```python
from build123d import *
from build123d.topology import SkipClean

# Parameters (mm, degrees)
CROQUIS1_R                   = 101.6
CROQUIS1_R_2                 = 7.9375
SALIENTE_EXTRUIR1_DEPTH      = 29
REDONDEO1_R                  = 28
CROQUIS2_R                   = 44.45
CORTAR_EXTRUIR1_DEPTH        = 8
CHAFL_N1_SIZE                = 15
CHAFL_N1_SIZE2               = 7.975641475
CHAFL_N2_SIZE                = 7.975641475
CHAFL_N2_SIZE_2              = 15
CORTAR_EXTRUIR2_DEPTH        = 147.581445076
CORTAR_EXTRUIR2_DEPTH_BACK   = 147.581445076
CROQUIS5_R                   = 7.9375
SALIENTE_EXTRUIR2_DEPTH      = 120
CROQUIS6_R                   = 12.9375
CROQUIS6_R_2                 = 7.9375
SALIENTE_EXTRUIR3_DEPTH      = 20
CROQUIS8_R                   = 3
CORTAR_EXTRUIR3_DEPTH        = 20
SALIENTE_EXTRUIR4_DEPTH      = 10
REDONDEO2_R                  = 1
CROQUIS11_R                  = 15
CORTAR_EXTRUIR4_DEPTH        = 50
SALIENTE_EXTRUIR5_DEPTH      = 5
SALIENTE_EXTRUIR5_DEPTH_BACK = 50
CROQUIS12_R                  = 15
CROQUIS12_R_2                = 7.9375
CROQUIS15_R                  = 7.9375
SALIENTE_EXTRUIR7_DEPTH      = 5
CROQUIS13_R                  = 3
SALIENTE_EXTRUIR8_DEPTH      = 5
SALIENTE_EXTRUIR8_2_DEPTH    = 5
SALIENTE_EXTRUIR8_3_DEPTH    = 5
SALIENTE_EXTRUIR8_4_DEPTH    = 5
CROQUIS17_R                  = 3
CORTAR_EXTRUIR5_DEPTH        = 16


with BuildPart() as part:
    # Croquis1 → Saliente-Extruir1 (new, symmetric)
    with BuildSketch(Plane.XY):
        with Locations(Location((0, 0, 0), (0, 0, 180))):
            Circle(CROQUIS1_R)
        with Locations(Location((0, 0, 0), (0, 0, 180))):
            Circle(CROQUIS1_R_2, mode=Mode.SUBTRACT)
    extrude(amount=SALIENTE_EXTRUIR1_DEPTH, both=True)

    # Redondeo1
    redondeo1_edges = [part.edges().sort_by_distance(p)[0] for p in [
        (101.6, 0, -29),
        (101.6, 0, 29),
    ]]
    fillet(redondeo1_edges, radius=REDONDEO1_R)

    # Croquis2 → Cortar-Extruir1 (cut)
    with BuildSketch(Plane(origin=(0, 0, -29), x_dir=(-1, 0, 0), z_dir=(0, 0, -1))):
        Circle(CROQUIS2_R)
    cortar_extruir1 = extrude(amount=-CORTAR_EXTRUIR1_DEPTH, mode=Mode.SUBTRACT)

    # Simetría3: Cortar-Extruir1 across plane
    add(cortar_extruir1.mirror(Plane.XY), mode=Mode.SUBTRACT)

    # Chaflán1
    chafl_n1_edges = [part.edges().sort_by_distance(p)[0] for p in [
        (44.45, 0, -29),
    ]]
    chafl_n1_side = [part.faces().sort_by_distance(p)[0] for p in [
        (71.518277636, 0, -29),
    ]]
    chamfer(chafl_n1_edges, length=CHAFL_N1_SIZE, length2=CHAFL_N1_SIZE2, reference=chafl_n1_side[0])

    # Chaflán2
    # the kernel refuses this chamfer: 15, 7.975641475 mm, written as the material it takes off along each edge
    with BuildSketch(Plane(origin=(0, 0, 29), x_dir=(-1, 0, 0), z_dir=(0, -1, 0))) as chafl_n2_piece_1_section:
        Polygon((44.45 + CHAFL_N2_SIZE, 0), (44.45, CHAFL_N2_SIZE_2), (44.45, 0), align=None)
    chafl_n2_piece_1 = revolve(axis=Axis((0, 0, 29), (0, 0, -1)), mode=Mode.PRIVATE)
    chafl_n2_piece_1 = split(chafl_n2_piece_1, bisect_by=Plane(origin=(50.219175815, 0, 21), z_dir=(0, 0, 1)), keep=Keep.TOP, mode=Mode.PRIVATE)
    add(chafl_n2_piece_1, mode=Mode.SUBTRACT)

    # Croquis3 → Cortar-Extruir2 (cut, two sides: drawn at the far end of the back side and taken through both)
    with BuildSketch(Plane(origin=(0, 0, 0), x_dir=(0, 0, -1), z_dir=(1, 0, 0)).offset(-CORTAR_EXTRUIR2_DEPTH_BACK)):
        Polygon((0, -580.951086966), (0, -121.331484358), (0, 121.331484358), (0, 580.951086966), (-919.239205217, 580.951086966), (-919.239205217, -580.951086966), align=None)
    extrude(amount=CORTAR_EXTRUIR2_DEPTH + CORTAR_EXTRUIR2_DEPTH_BACK, mode=Mode.SUBTRACT)

    # Simetría4: part across plane


with BuildPart() as part_1:
    add(part.part)
    add(part.part.mirror(Plane(origin=(376.375487344, -121.331484358, 0), x_dir=(1, 0, 0), z_dir=(0, 0, 1))))

    # Croquis11 → Cortar-Extruir4 (cut)
    with BuildSketch(Plane.XY.offset(21)):
        Circle(CROQUIS11_R)
    extrude(amount=-CORTAR_EXTRUIR4_DEPTH, mode=Mode.SUBTRACT)


with BuildPart() as body_2:
    # Croquis5 → Saliente-Extruir2 (new body)
    with BuildSketch(Plane.XY.offset(21)):
        with Locations(Location((0, 0, 0), (0, 0, 180))):
            Circle(CROQUIS5_R)
    extrude(amount=-SALIENTE_EXTRUIR2_DEPTH)


with BuildPart() as body_3:
    # Croquis6 → Saliente-Extruir3 (new body)
    with BuildSketch(Plane(origin=(0, 0, -99), x_dir=(-1, 0, 0), z_dir=(0, 0, -1))):
        Circle(CROQUIS6_R)
        Circle(CROQUIS6_R_2, mode=Mode.SUBTRACT)
    extrude(amount=-SALIENTE_EXTRUIR3_DEPTH)

    # Croquis8 → Cortar-Extruir3 (cut)
    with BuildSketch(Plane(origin=(0, 0, 0), x_dir=(1, 0, 0), z_dir=(0, 1, 0))):
        with Locations(Location((0, 89, 0), (0, 0, 90))):
            Circle(CROQUIS8_R)
    extrude(amount=CORTAR_EXTRUIR3_DEPTH, mode=Mode.SUBTRACT)

    # Croquis10 → Saliente-Extruir4 (add)
    with BuildSketch(Plane(origin=(0, 0, -99), x_dir=(-1, 0, 0), z_dir=(0, 0, -1))):
        with BuildLine():
            Line((-5, 17.5), (5, 17.5))
            ThreePointArc((5, 17.5), (7.856559563, 13.607960336), (12.655444566, 13.080127019))
            Line((12.655444566, 13.080127019), (17.655444566, 4.419872981))
            ThreePointArc((17.655444566, 4.419872981), (15.713119126, 0), (17.655444566, -4.419872981))
            Line((17.655444566, -4.419872981), (12.655444566, -13.080127019))
            ThreePointArc((12.655444566, -13.080127019), (7.856559563, -13.607960336), (5, -17.5))
            Line((5, -17.5), (-5, -17.5))
            ThreePointArc((-5, -17.5), (-7.856559563, -13.607960336), (-12.655444566, -13.080127019))
            Line((-12.655444566, -13.080127019), (-17.655444566, -4.419872981))
            ThreePointArc((-17.655444566, -4.419872981), (-15.713119126, 0), (-17.655444566, 4.419872981))
            Line((-17.655444566, 4.419872981), (-12.655444566, 13.080127019))
            ThreePointArc((-12.655444566, 13.080127019), (-7.856559563, 13.607960336), (-5, 17.5))
        make_face()
    extrude(amount=SALIENTE_EXTRUIR4_DEPTH)

    # Redondeo2
    redondeo2_edges = [body_3.edges().sort_by_distance(p)[0] for p in [
        (5, 17.5, -104),
        (12.655444566, 13.080127019, -104),
        (17.655444566, 4.419872981, -104),
        (17.655444566, -4.419872981, -104),
        (12.655444566, -13.080127019, -104),
        (5, -17.5, -104),
        (-5, -17.5, -104),
        (-12.655444566, -13.080127019, -104),
        (-17.655444566, -4.419872981, -104),
        (-17.655444566, 4.419872981, -104),
        (-12.655444566, 13.080127019, -104),
        (-5, 17.5, -104),
    ]]
    fillet(redondeo2_edges, radius=REDONDEO2_R)


with BuildPart() as body_4:
    # Croquis12 → Saliente-Extruir5 (new, two sides: drawn at the far end of the back side and taken through both)
    with BuildSketch(Plane.XY.offset(21).offset(-SALIENTE_EXTRUIR5_DEPTH_BACK)):
        Circle(CROQUIS12_R)
        with Locations(Location((0, 0, 0), (0, 0, 180))):
            Circle(CROQUIS12_R_2, mode=Mode.SUBTRACT)
    extrude(amount=SALIENTE_EXTRUIR5_DEPTH + SALIENTE_EXTRUIR5_DEPTH_BACK)


with BuildPart() as body_5:
    # Croquis15 → Saliente-Extruir7 (new body)
    with BuildSketch(Plane.XY.offset(21)):
        with Locations(Location((0, 0, 0), (0, 0, 180))):
            Circle(CROQUIS15_R)
    extrude(amount=SALIENTE_EXTRUIR7_DEPTH)

    # Combinar1: union body 2
    add(body_2.part)


with BuildPart() as body_5_2:
    # Croquis13 → Saliente-Extruir8 (new body)
    with BuildSketch(Plane.XY.offset(26)):
        with BuildLine():
            Line((5, -25), (5, -6.164730834))
            ThreePointArc((5, -6.164730834), (0, -7.9375), (-5, -6.164730834))
            Line((-5, -6.164730834), (-5, -25))
            Line((-5, -25), (5, -25))
        make_face()
        with Locations((0, -18.5)):
            Circle(CROQUIS13_R, mode=Mode.SUBTRACT)
    extrude(amount=-SALIENTE_EXTRUIR8_DEPTH)


with BuildPart() as body_6:
    # Croquis13 → Saliente-Extruir8 2 (new body)
    with BuildSketch(Plane.XY.offset(26)):
        with BuildLine():
            Line((-5, 25), (5, 25))
            Line((5, 25), (5, 6.164730834))
            ThreePointArc((5, 6.164730834), (0, 7.9375), (-5, 6.164730834))
            Line((-5, 6.164730834), (-5, 25))
        make_face()
        with Locations((0, 18.5)):
            Circle(CROQUIS13_R, mode=Mode.SUBTRACT)
    extrude(amount=-SALIENTE_EXTRUIR8_2_DEPTH)


with BuildPart() as body_7:
    # Croquis13 → Saliente-Extruir8 3 (new body)
    with BuildSketch(Plane.XY.offset(26)):
        with BuildLine():
            Line((-25, -5), (-6.164730834, -5))
            ThreePointArc((-6.164730834, -5), (-7.9375, 0), (-6.164730834, 5))
            Line((-6.164730834, 5), (-25, 5))
            Line((-25, 5), (-25, 0))
            Line((-25, 0), (-25, -5))
        make_face()
        with Locations((-18.5, 0)):
            Circle(CROQUIS13_R, mode=Mode.SUBTRACT)
    extrude(amount=-SALIENTE_EXTRUIR8_3_DEPTH)


with BuildPart() as body_8:
    # Croquis13 → Saliente-Extruir8 4 (new body)
    with BuildSketch(Plane.XY.offset(26)):
        with BuildLine():
            Line((25, -5), (25, 5))
            Line((25, 5), (6.164730834, 5))
            ThreePointArc((6.164730834, 5), (7.9375, 0), (6.164730834, -5))
            Line((6.164730834, -5), (25, -5))
        make_face()
        with Locations((18.5, 0)):
            Circle(CROQUIS13_R, mode=Mode.SUBTRACT)
    extrude(amount=-SALIENTE_EXTRUIR8_4_DEPTH)


with BuildPart() as body_4_1:
    add(body_4.part)

    # Combinar2: union body 6, body 8, body 5 2, body 7
    add(body_6.part)
    add(body_8.part)
    add(body_5_2.part)
    add(body_7.part)

    # Croquis17 → Cortar-Extruir5 (cut)
    with SkipClean():  # the faces are left unmerged after this step: merging them gives an invalid solid
        with BuildSketch(Plane(origin=(0, 0, 0), x_dir=(1, 0, 0), z_dir=(0, 1, 0))):
            with Locations(Location((0, 24, 0), (0, 0, 90))):
                Circle(CROQUIS17_R)
        extrude(amount=CORTAR_EXTRUIR5_DEPTH, mode=Mode.SUBTRACT)


solid = part_1.part
```
Model file for the job. Use its own axes, mm. A direction names the side the tool comes from. Coordinates: 2 decimals unless noted, no trailing zeros. Loops run counter-clockwise (first coordinate to the right, second up) from the corner with the lowest first, then second, coordinate; pieces in that order, holes last. Notation, with made-up numbers: M -23.75,21 L 29.25,21 A28 cw 29.25,43 Z; hole C 12,67.5 d4. An arc over 180 degrees is marked long. Use CSV: the item, a comma, the result in double quotes. Start each with the question number.
1. Band-saw the part on C-C, the plane z = 7.5. List the corners of the cut face in (x, y), then the cut area to 3 significant figures.
2. Probe probe 1 along X at (y, z) = (28, 25); probe 2 along Z at (x, y) = (-28, -13); probe 3 along Y at (x, z) = (0, -20.95). List the from-to ranges inside material, lowest first. Write a range as [from, to].
3. Flat gauge pins, fed straight in: pin 1 (2 mm diameter, centred on x = 48.5, z = -13.5, fed in from -Y); pin 2 (1.5 mm diameter, centred on x = 59.5, y = 55.5, fed in from -Z); pin 3 (8 mm diameter, centred on x = 43, y = 78, fed in from +Z); pin 4 (18 mm diameter, centred on x = 0, y = 0, fed in from -Z). Where does each tip first touch, or does it go through?
4. Tool access for faces 4 (the flat face through (1, -19, 21)), 5 (the conical face through (9.79, -44.1, -21.41)): list every direction of +Z, -Z, +X, -X, +Y, -Y with a clear straight run to the whole face (end or side of a thin tool).
5. Two-plate mould, pull along Y, no slides. Class faces 1 (the flat face through (1, -19, -21)), 2 (the flat face through (-60, 0, 29)), 3 (the cylindrical face through (-14.985, 0.66, 0.294)): pulls with the +Y half, pulls with the -Y half, needs draft (parallel to the pull), parting line crosses it, or undercut.
Entries:
1,outline,"C 0,0 d201.67; hole C 0,0 d30"
1,area,"31,200 mm2"
2,probe 1,"x = [-83.45, -43.73], [43.73, 83.45]"
2,probe 2,"z = [-21, 21]"
2,probe 3,"y = [-93.25, -15], [15, 93.25]"
3,pin 1,"stops at y = -86.69"
3,pin 2,"stops at z = -28.11"
3,pin 3,"stops at z = 26.54"
3,pin 4,"passes through"
4,face 4,"+Z"
4,face 5,"-Z"
5,face 1,"undercut"
5,face 2,"needs draft"
5,face 3,"undercut"
